```python
from build123d import *

# Parameters (mm, degrees)
SKETCH1_W           = 40
SKETCH1_H           = 25
SKETCH1_R           = 1.5
BOSS_EXTRUDE1_DEPTH = 3
SKETCH2_W           = 2
SKETCH2_H           = 10
BOSS_EXTRUDE2_DEPTH = 75
SKETCH6_W           = 25
SKETCH6_H           = 35
BOSS_EXTRUDE3_DEPTH = 2.5
SKETCH7_W           = 35
SKETCH7_H           = 2.5
BOSS_EXTRUDE4_DEPTH = 12.5
SKETCH8_W           = 5
SKETCH8_H           = 46
CUT_EXTRUDE2_DEPTH  = 90.862394805


with BuildPart() as part:
    # Sketch1 → Boss-Extrude1 (new body)
    with BuildSketch(Plane(origin=(0, 0, 0), x_dir=(1, 0, 0), z_dir=(0, 1, 0))):
        with Locations((-20, 12.5)):
            Rectangle(SKETCH1_W, SKETCH1_H)
        with Locations(Location((-5.5, 20.7, 0), (0, 0, 270))):
            Circle(SKETCH1_R, mode=Mode.SUBTRACT)
        with Locations(Location((-5.5, 4.3, 0), (0, 0, 270))):
            Circle(SKETCH1_R, mode=Mode.SUBTRACT)
    extrude(amount=BOSS_EXTRUDE1_DEPTH)

    # Sketch2 → Boss-Extrude2 (add)
    with BuildSketch(Plane.XZ):
        with Locations((-39, -20)):
            Rectangle(SKETCH2_W, SKETCH2_H)
    extrude(amount=BOSS_EXTRUDE2_DEPTH)

    # Sketch6 → Boss-Extrude3 (add)
    with BuildSketch(Plane.XZ.offset(75)):
        with Locations((-27.5, -7.5)):
            Rectangle(SKETCH6_W, SKETCH6_H)
    extrude(amount=BOSS_EXTRUDE3_DEPTH)

    # Sketch7 → Boss-Extrude4 (add)
    with BuildSketch(Plane(origin=(-38, 0, 0), x_dir=(0, 0, -1), z_dir=(1, 0, 0))):
        with Locations((7.5, -23.75)):
            Rectangle(SKETCH7_W, SKETCH7_H)
    extrude(amount=BOSS_EXTRUDE4_DEPTH)

    # Sketch8 → Cut-Extrude2 (cut, through all)
    with BuildSketch(Plane(origin=(-38, 0, 0), x_dir=(0, 0, -1), z_dir=(1, 0, 0))):
        with Locations((17.5, -50)):
            Rectangle(SKETCH8_W, SKETCH8_H)
    extrude(amount=-CUT_EXTRUDE2_DEPTH, mode=Mode.SUBTRACT)


solid = part.part
```
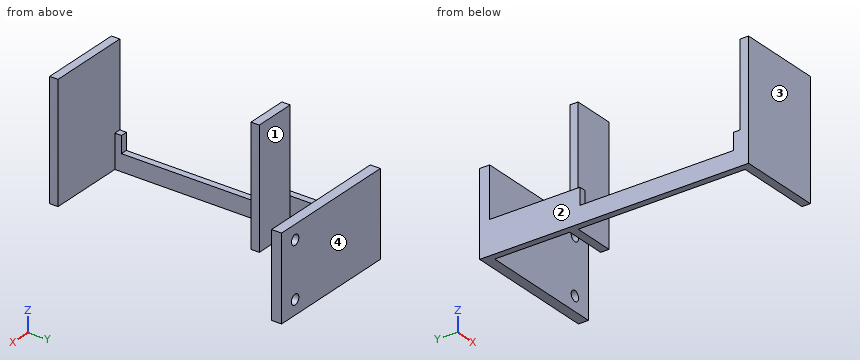
Could you check a few things on this model? Use its own coordinates, in mm. Face numbers are marked on the shaded views. Round coordinates to 2 decimals unless told otherwise and drop trailing zeros. Loops run counter-clockwise (first coordinate to the right, second up) from the corner with the lowest first, then second, coordinate; pieces in that order, holes last. Notation, with made-up numbers: M 35,-7 L 50,-7 A36 cw 50,27 Z; hole C 5.25,17.5 d9. An arc over 180 degrees is marked long. Put each result on its own line as item: value.
Q1. Imagine slicing it at B-B (x = -23). Write out the boundary of the cut face in (y, z), then the cut area to 4 significant figures.
Check result:
outline: M -77.5,-25 L -75,-25 L -75,10 L -77.5,10 Z; M 0,-25 L 3,-25 L 3,0 L 0,0 Z
area: 162.5 mm2
Q2. I need wall thicknesses on probe 1 along Y at (x, z) = (-30, -2); probe 2 along Y at (x, z) = (-24, -2); probe 3 along X at (y, z) = (2.2, -20.7). Which ranges of each line are inside material? Lowest first, please.
Check result:
probe 1: -77.5 to -75, -25 to -22.5, 0 to 3
probe 2: -77.5 to -75, 0 to 3
probe 3: -40 to -7, -4 to 0
Q3. Imagine slicing it at C-C (x = -32.5). Write out the boundary of the cut face in (y, z).
Check result:
outline: M -77.5,-25 L -75,-25 L -75,10 L -77.5,10 Z; M -25,-25 L -22.5,-25 L -22.5,10 L -25,10 Z; M 0,-25 L 3,-25 L 3,0 L 0,0 Z
Q4. Thinking about a two-plate mould opening in Y: for the marked faces 1, 2, 3 and 4, which applies, released by +Y, released by -Y, zero draft, split by the parting line, or undercut?
Check result:
face 1: undercut
face 2: zero draft
face 3: released by -Y
face 4: released by +Y
Q5. Imagine slicing it at A-A (z = -1). Write out the boundary of the cut face in (x, y).
Check result:
outline: M -40,-77.5 L -15,-77.5 L -15,-75 L -40,-75 Z; M -40,0 L 0,0 L 0,3 L -40,3 Z; M -38,-25 L -25.5,-25 L -25.5,-22.5 L -38,-22.5 Z
Q6. Imagine slicing it at D-D (z = -5). Write out the boundary of the cut face in (x, y).
Check result:
outline: M -40,-77.5 L -15,-77.5 L -15,-75 L -40,-75 Z; M -40,0 L -6.83,0 L -6.83,3 L -40,3 Z; M -38,-25 L -25.5,-25 L -25.5,-22.5 L -38,-22.5 Z; M -4.17,0 L 0,0 L 0,3 L -4.17,3 Z
Q7. For pin 1 (2.5 mm diameter, centred on x = -5.5, z = -20.7, fed in from +Y); pin 2 (11 mm diameter, centred on y = -15, z = -21.5, fed in from +X); pin 3 (2 mm diameter, centred on y = -76.5, z = -6, fed in from +X); pin 4 (1.6 mm diameter, centred on x = -39, y = -49, fed in from +Z), each with a flat end and sliding along its axis, tell me the tip position at first contact or that it passes through.
Check result:
pin 1: through
pin 2: x = -38
pin 3: x = -15
pin 4: z = -20
